from build123d import *

# Parameters (mm, degrees)
SKETCH1_R           = 1.6
BOSS_EXTRUDE1_DEPTH = 3
SKETCH3_R           = 1.5
SKETCH3_R_2         = 5
CUT_EXTRUDE2_DEPTH  = 4
FILLET1_R           = 10


with BuildPart() as part:
    # Sketch1 → Boss-Extrude1 (new body)
    with BuildSketch(Plane(origin=(0, 0, 0), x_dir=(1, 0, 0), z_dir=(0, 1, 0))):
        Polygon((-31.529631255, 126.118525019), (31.529631255, 126.118525019), (124.986662182, -35.753800871), (93.457030927, -90.364724148), (-93.457030927, -90.364724148), (-124.986662182, -35.753800871), align=None)
        with Locations((-25, 115)):
            Circle(SKETCH1_R, mode=Mode.SUBTRACT)
        with Locations((-12.009618943, 92.5)):
            Circle(SKETCH1_R, mode=Mode.SUBTRACT)
        with Locations((-37.990381057, 92.5)):
            Circle(SKETCH1_R, mode=Mode.SUBTRACT)
        with Locations((37.990381057, 92.5)):
            Circle(SKETCH1_R, mode=Mode.SUBTRACT)
        with Locations((12.009618943, 92.5)):
            Circle(SKETCH1_R, mode=Mode.SUBTRACT)
        with Locations((25, 115)):
            Circle(SKETCH1_R, mode=Mode.SUBTRACT)
        with Locations((112.092921435, -35.849364905)):
            Circle(SKETCH1_R, mode=Mode.SUBTRACT)
        with Locations((86.112159322, -35.849364905)):
            Circle(SKETCH1_R, mode=Mode.SUBTRACT)
        with Locations((99.102540378, -13.349364905)):
            Circle(SKETCH1_R, mode=Mode.SUBTRACT)
        with Locations((74.102540378, -56.650635095)):
            Circle(SKETCH1_R, mode=Mode.SUBTRACT)
        with Locations((87.092921435, -79.150635095)):
            Circle(SKETCH1_R, mode=Mode.SUBTRACT)
        with Locations((61.112159322, -79.150635095)):
            Circle(SKETCH1_R, mode=Mode.SUBTRACT)
        with Locations((-87.092921435, -79.150635095)):
            Circle(SKETCH1_R, mode=Mode.SUBTRACT)
        with Locations((-74.102540378, -56.650635095)):
            Circle(SKETCH1_R, mode=Mode.SUBTRACT)
        with Locations((-61.112159322, -79.150635095)):
            Circle(SKETCH1_R, mode=Mode.SUBTRACT)
        with Locations((-86.112159322, -35.849364905)):
            Circle(SKETCH1_R, mode=Mode.SUBTRACT)
        with Locations((-112.092921435, -35.849364905)):
            Circle(SKETCH1_R, mode=Mode.SUBTRACT)
        with Locations((-99.102540378, -13.349364905)):
            Circle(SKETCH1_R, mode=Mode.SUBTRACT)
    extrude(amount=BOSS_EXTRUDE1_DEPTH)

    # Sketch3 → Cut-Extrude2 (cut, through all)
    with BuildSketch(Plane(origin=(0, 3, 0), x_dir=(1, 0, 0), z_dir=(0, 1, 0))):
        with Locations((-12.5, 12.5)):
            Circle(SKETCH3_R)
        with Locations((12.5, 12.5)):
            Circle(SKETCH3_R)
        with Locations((12.5, -12.5)):
            Circle(SKETCH3_R)
        with Locations((-12.5, -12.5)):
            Circle(SKETCH3_R)
        with Locations((-50, 28.867513459)):
            Circle(SKETCH3_R_2)
        with Locations((50, 28.867513459)):
            Circle(SKETCH3_R_2)
        with Locations((0, -57.735026919)):
            Circle(SKETCH3_R_2)
        Circle(SKETCH3_R_2)
    extrude(amount=-CUT_EXTRUDE2_DEPTH, mode=Mode.SUBTRACT)

    # Fillet1
    fillet1_edges = [part.edges().sort_by_distance(p)[0] for p in [
        (-31.529631255, 1.5, -126.118525019),
        (31.529631255, 1.5, -126.118525019),
        (124.986662182, 1.5, 35.753800871),
        (93.457030927, 1.5, 90.364724148),
        (-93.457030927, 1.5, 90.364724148),
        (-124.986662182, 1.5, 35.753800871),
    ]]
    fillet(fillet1_edges, radius=FILLET1_R)


solid = part.part
Read the model definition and answer for the solid it produces. Units are mm, in the model's axes. Give positions to 0.01 mm unless a question says otherwise; leave off trailing zeros. Write each loop counter-clockwise with the first axis right and the second up, starting at its lowest first coordinate (ties: lowest second). Pieces come first, ordered by that corner, then holes. Notation, with made-up numbers: (82, 1.5) - (102, 1.5) arc R12 cw to (102, 15.5) - close; hole circle Ø2 at (-26, 9.25). An arc over 180 degrees is marked (long way). Answer in a Markdown table with one row per item. Add a question column.
Item 1: Section C-C, the plane y = 2.4 is taken. Count the separate pieces of the cut face and the enclosed holes in it, and give its area (3 significant figures).
Item 2: Section B-B, the plane x = 50 is taken. Write down the section's boundary in (y, z).
Item 3: Section D-D, the plane z = -84 is taken. Write down the section's boundary in (x, y).
Item 4: Find the intervals of material crossed by L1, parallel to X at y = 2.35, z = 79; L2, parallel to Z at x = -25, y = 1.5; L3, parallel to X at y = 2.8, z = -114.5, in increasing order.
Item 5: Section A-A, the plane x = 0 is taken. Write down the section's boundary in (y, z).
Item 6: Determine the mould class of faces 1 (the face through (92.747, 1.521, 88.988)), 2 (the face through (45, 2, -29)), 3 (the face through (2, 0, -19)) for opening direction Z: pulls with the +Z half, pulls with the -Z half, needs draft (parallel to the pull), parting line crosses it, or undercut.
Recorded:
| question | item | result |
|---|---|---|
| 1 | separate pieces | 1 |
| 1 | enclosed holes | 26 |
| 1 | area | 36,700 mm2 |
| 2 | outline | (0, -94.13) - (3, -94.13) - (3, -33.87) - (0, -33.87) - close; (0, -23.87) - (3, -23.87) - (3, 90.36) - (0, 90.36) - close |
| 3 | outline | (-55.85, 0) - (55.85, 0) - (55.85, 3) - (-55.85, 3) - close |
| 4 | L1 | x = -100.02 to -88.69, -85.5 to -62.71, -59.52 to 59.52, 62.71 to 85.5, 88.69 to 100.02 |
| 4 | L2 | z = -126.12 to -116.6, -113.4 to 90.36 |
| 4 | L3 | x = -38.24 to -26.52, -23.48 to 23.48, 26.52 to 38.24 |
| 5 | outline | (0, -126.12) - (3, -126.12) - (3, -5) - (0, -5) - close; (0, 5) - (3, 5) - (3, 52.74) - (0, 52.74) - close; (0, 62.74) - (3, 62.74) - (3, 90.36) - (0, 90.36) - close |
| 6 | face 1 | pulls with the +Z half |
| 6 | face 2 | undercut |
| 6 | face 3 | needs draft |
